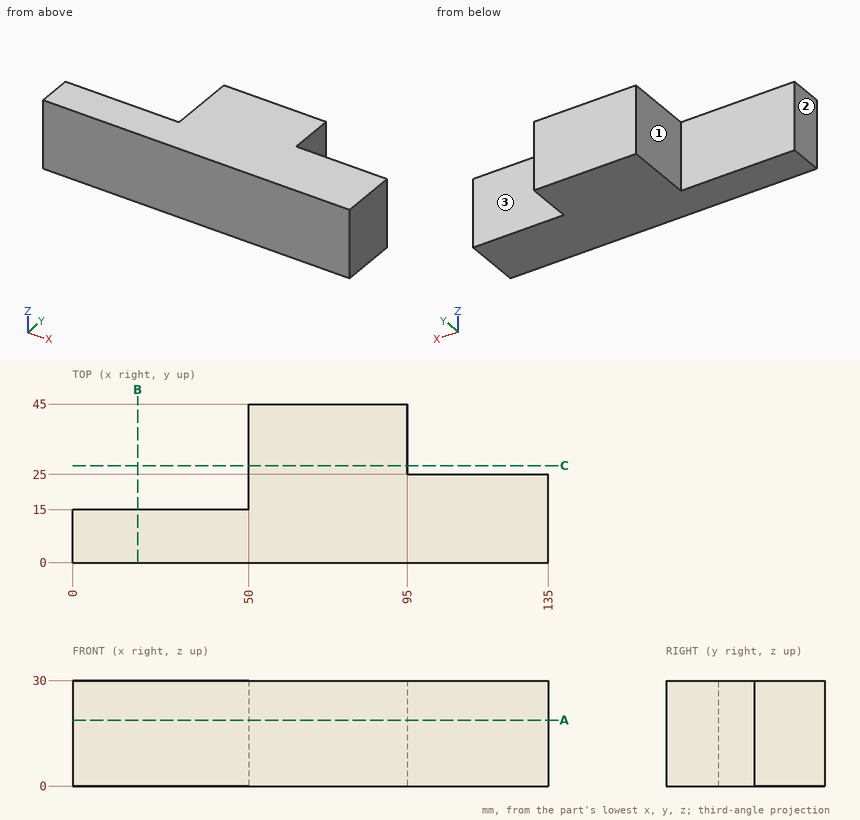
Input: dimensioned drawing with shaded views. Units: mm. Origin: part minimum x, y, z. A direction names the side the tool comes from. Coordinates: 2 decimals unless noted, no trailing zeros. Loops run counter-clockwise (first coordinate to the right, second up) from the corner with the lowest first, then second, coordinate; pieces in that order, holes last.
Q1. Set-up query: the marked faces 1, 2 and 3. Return all of +Z, -Z, +X, -X, +Y, -Y with unobstructed straight access to the full face (end or side cutting, diameter ignored); none if empty.
Results are:
face 1: +Z, -Z, -X, +Y
face 2: +Z, -Z, -X, +Y, -Y
face 3: +Z, -Z, +X, +Y
Q2. Line query: line 1 along X through (y, z) = (17, 14.75); line 2 along Y through (x, z) = (43, 2); line 3 along X through (y, z) = (41.5, 12.25). Output: solid intervals per line, ascending.
Results are:
line 1: x = 50 to 135
line 2: y = 0 to 15
line 3: x = 50 to 95
Q3. Section B-B, the plane x = 18.5. Return the cut outline in (y, z).
Results are:
outline: (0, 0) - (15, 0) - (15, 30) - (0, 30) - close
Q4. Section A-A, the plane z = 18.75. Return the cut outline in (x, y).
Results are:
outline: (0, 0) - (135, 0) - (135, 25) - (95, 25) - (95, 45) - (50, 45) - (50, 15) - (0, 15) - close
Q5. Contact query for flat-ended pins moving along their axis: pin 1 (5 mm diameter, centred on x = 38, z = 18.5, fed in from +Y); pin 2 (8 mm diameter, centred on x = 117.5, z = 7.5, fed in from +Y); pin 3 (1 mm diameter, centred on y = 40, z = 3.5, fed in from -X). Output: stop coordinate, or through.
Results are:
pin 1: stops at y = 15
pin 2: stops at y = 25
pin 3: stops at x = 50
Q6. Section C-C, the plane y = 27.5. Return the cut outline in (x, z).
Results are:
outline: (50, 0) - (95, 0) - (95, 30) - (50, 30) - close
